```python
from build123d import *

# Parameters (mm, degrees)
F0_W     = 600
F0_H     = 850
F0_W_2   = 570
F0_H_2   = 820
F1_DEPTH = 20
F2_W     = 600
F2_H     = 850
F3_DEPTH = 5


with BuildPart() as f1:
    # F0 (on Front) → F1 (new body)
    with BuildSketch(Plane.XZ):
        with Locations((260.588973, 360.083479)):
            Rectangle(F0_W, F0_H)
        with Locations((260.588973, 360.083479)):
            Rectangle(F0_W_2, F0_H_2, mode=Mode.SUBTRACT)
    extrude(amount=F1_DEPTH)

    # F2 (on face) → F3 (join)
    with BuildSketch(Plane.XZ.offset(20)):
        with Locations((260.588973, 360.083479)):
            Rectangle(F2_W, F2_H)
    extrude(amount=-F3_DEPTH)


solid = f1.part
```
Check sheet for the modelled part. Datum: model origin and axes. Units: mm. Round coordinates to 2 decimals unless told otherwise and drop trailing zeros. Write each loop counter-clockwise with the first axis right and the second up, starting at its lowest first coordinate (ties: lowest second). Pieces come first, ordered by that corner, then holes. Notation, with made-up numbers: (-38, -5) -> (10, -5) arc R23 cw to (10, 18) -> close; hole circle Ø1 at (-19, 46.5). An arc over 180 degrees is marked (long way). Put each result on its own line as item: value.
(1) Material ranges on line 1 (Z direction, x = 416.5, y = -2); line 2 (X direction, y = -7.5, z = 553.5); line 3 (Y direction, x = 29.5, z = 709), recorded low to high.
Values found:
line 1: z = -64.92 to -49.92, 770.08 to 785.08
line 2: x = -39.41 to -24.41, 545.59 to 560.59
line 3: y = -20 to -15
(2) Go/stop test with a flat-tipped pin: pin 1 Ø3 at (x, z) = (90, 479.5) entering from +Y. Record where the tip stops, or that it passes through.
Values found:
pin 1: stops at y = -15
(3) Sectioned sample at C-C (x = 265). Enter the section's corners in (y, z).
Values found:
outline: (-20, -64.92) -> (0, -64.92) -> (0, -49.92) -> (-15, -49.92) -> (-15, 770.08) -> (0, 770.08) -> (0, 785.08) -> (-20, 785.08) -> close
(4) Mould release check, pull along X, two halves, no side actions. Record for faces 1 (the face through (256, -10, 785.083)), 2 (the face through (-39.411, -10, 354)), 3 (the face through (257, -15, 366)): released by +X, released by -X, zero draft, split by the parting line, or undercut.
Values found:
face 1: zero draft
face 2: released by -X
face 3: undercut
(5) Sectioned sample at A-A (y = -3). Enter the section's corners in (x, z).
Values found:
outline: (-39.41, -64.92) -> (560.59, -64.92) -> (560.59, 785.08) -> (-39.41, 785.08) -> close; hole (-24.41, -49.92) -> (545.59, -49.92) -> (545.59, 770.08) -> (-24.41, 770.08) -> close
(6) Sectioned sample at B-B (z = 408.5). Enter the section's corners in (x, y).
Values found:
outline: (-39.41, -20) -> (560.59, -20) -> (560.59, 0) -> (545.59, 0) -> (545.59, -15) -> (-24.41, -15) -> (-24.41, 0) -> (-39.41, 0) -> close
